Autodesk Inventor part; units mm, degrees
ref_plane "YZ Plane" through (0, 0, 0) normal (1, 0, 0) x (0, 1, 0)
ref_plane "XZ Plane" through (0, 0, 0) normal (0, 1, 0) x (-1, 0, 0)
ref_plane "XY Plane" through (0, 0, 0) normal (0, 0, 1) x (1, 0, 0)
sketch "Sketch1" plane through (0, 0, 0) normal (0, 0, 1) x (1, 0, 0)
  line L0 (-2.735, 4.7371) -> (2.735, 4.7371)
  line L1 (2.735, 4.7371) -> (5.4699, 0)
  line L2 (5.4699, 0) -> (2.735, -4.7371)
  line L3 (2.735, -4.7371) -> (-2.735, -4.7371)
  line L4 (-2.735, -4.7371) -> (-5.4699, 0)
  line L5 (-5.4699, 0) -> (-2.735, 4.7371)
  point P0 (0, 0)
  point P1 (0, 0)
  dimension "d0" = 9.4742
extrude "Extrusion1" add sketch "Sketch1" along normal mid plane 62.992
sketch "Sketch2" plane through (0, 0, 31.496) normal (0, 0, 1) x (1, 0, 0)
  circle A0 centre (0, 0) radius 4.7371
  dimension "d3" = 9.4742
extrude "Extrusion2" add sketch "Sketch2" along normal blind 4.445
sketch "Sketch3" plane through (0, 0, -31.496) normal (0, 0, -1) x (-1, 0, 0)
  circle A0 centre (0, 0) radius 4.7371
  dimension "d6" = 9.4742
extrude "Extrusion3" add sketch "Sketch3" along normal blind 4.445
properties part number "AM shifter new input shaft" material "Steel"
Check sheet for the modelled part. Datum: model origin and axes. Units: mm. A direction names the side the tool comes from. Coordinates: 2 decimals unless noted, no trailing zeros. Loops run counter-clockwise (first coordinate to the right, second up) from the corner with the lowest first, then second, coordinate; pieces in that order, holes last. Notation, with made-up numbers: (64.5, -25) -> (94.5, -25) arc R19 ccw to (94.5, 10) -> close; hole circle Ø8 at (86, 82). An arc over 180 degrees is marked (long way). Write item = value, one per line. Start each with the question number.
1. Section check C-C on y = -3.5. Record the cut outline in (x, z).
2. Material ranges on line 1 (Z direction, x = -3, y = -4); line 2 (X direction, y = 2, z = -19); line 3 (X direction, y = 1, z = -12.5), recorded low to high.
3. Section check A-A on y = 1.5. Record the cut outline in (x, z).
4. Depth check by flat-ended pin: P1, Ø0.7, axis at x = -3, y = -4, coming from the -Z side; P2, Ø1.5, axis at y = 1, z = 11.5, coming from the -X side. Enter the tip coordinate at first touch or a pass-through.
5. Tool access check on faces 1 (the flat face through (2.5, -4.2, -31.496)), 2 (the flat face through (-2.4, 4.3, -31.496)), 3 (the flat face through (5, 0, 31.496)), 4 (the cylindrical face through (-1.027, 4.624, 33.687)), 5 (the flat face through (2.5, -4.2, 31.496)). Record the directions out of +Z, -Z, +X, -X, +Y, -Y that give a thin tool (end or side, any length) a straight path to the whole face; none if there is none.
6. Section check B-B on z = 8.5. Record the cut outline in (x, y) (3 decimals).
Responses:
q1.outline = (-3.45, -31.5) -> (-3.19, -31.5) -> (-3.19, -35.94) -> (3.19, -35.94) -> (3.19, -31.5) -> (3.45, -31.5) -> (3.45, 31.5) -> (3.19, 31.5) -> (3.19, 35.94) -> (-3.19, 35.94) -> (-3.19, 31.5) -> (-3.45, 31.5) -> close
q2.line_1 = -31.5 to 31.5
q2.line_2 = -4.32 to 4.32
q2.line_3 = -4.89 to 4.89
q3.outline = (-4.6, -31.5) -> (-4.49, -31.5) -> (-4.49, -35.94) -> (4.49, -35.94) -> (4.49, -31.5) -> (4.6, -31.5) -> (4.6, 31.5) -> (4.49, 31.5) -> (4.49, 35.94) -> (-4.49, 35.94) -> (-4.49, 31.5) -> (-4.6, 31.5) -> close
q4.P1 = -35.94
q4.P2 = -5.33
q5.face_1 = -Z, +X, -Y
q5.face_2 = -Z, -X, +Y
q5.face_3 = +Z, +X
q5.face_4 = +Z
q5.face_5 = +Z, +X, -Y
q6.outline = (-5.47, 0) -> (-2.735, -4.737) -> (2.735, -4.737) -> (5.47, 0) -> (2.735, 4.737) -> (-2.735, 4.737) -> close
